Autodesk Inventor part; units mm, degrees
ref_plane "YZ Plane" through (0, 0, 0) normal (1, 0, 0) x (0, 1, 0)
ref_plane "XZ Plane" through (0, 0, 0) normal (0, 1, 0) x (-1, 0, 0)
ref_plane "XY Plane" through (0, 0, 0) normal (0, 0, 1) x (1, 0, 0)
sketch "Esquisse1" plane through (0, 0, 0) normal (0, 1, 0) x (-1, 0, 0)
  line L0 (-32.5, 48.5) -> (32.5, 48.5)
  line L1 (32.5, 48.5) -> (32.5, -48.5)
  line L2 (32.5, -48.5) -> (-32.5, -48.5)
  line L3 (-32.5, -48.5) -> (-32.5, 48.5)
  point P0 (0, 0)
  dimension "d0" = 65
  dimension "d1" = 97
  dimension "d2" = 32.5
  dimension "d3" = 48.5
extrude "Extrusion1" add sketch "Esquisse1" along normal blind 1.5
sketch "Esquisse2" plane through (0, 1.5, 0) normal (0, 1, 0) x (1, 0, 0)
  line L0 (-32.5, -48.5) -> (32.5, -48.5)
  line L1 (32.5, -48.5) -> (32.5, 48.5)
  line L2 (-32.5, 48.5) -> (-32.5, -48.5)
  line L3 (-27.5, 17.5) -> (-22.5, 17.5)
  line L4 (-22.5, 17.5) -> (-22.5, -47.5)
  line L5 (-22.5, -47.5) -> (-27.5, -47.5)
  line L6 (-27.5, -47.5) -> (-27.5, 17.5)
  line L7 (22.5, 17.5) -> (27.5, 17.5)
  line L8 (27.5, 17.5) -> (27.5, -47.5)
  line L9 (27.5, -47.5) -> (22.5, -47.5)
  line L10 (22.5, -47.5) -> (22.5, 17.5)
  point P0 (0, 0)
  dimension "d6" = 5
  dimension "d7" = 5
  dimension "d8" = 65
  dimension "d9" = 5
  dimension "d10" = 5
  dimension "d11" = 1
extrude "Extrusion2" add sketch "Esquisse2" along normal blind 9 and the other way blind 5.5
sketch "Esquisse3" plane through (0, 0, 0) normal (0, -1, 0) x (1, 0, 0)
  line L0 (32.5, 48.5) -> (-32.5, 48.5)
  line L1 (32.5, -48.5) -> (32.5, 48.5)
  line L2 (9.5, 48.5) -> (17.5, 48.5)
  line L3 (17.5, 48.5) -> (17.5, 33.5)
  line L4 (17.5, 33.5) -> (9.5, 33.5)
  line L5 (9.5, 33.5) -> (9.5, 48.5)
  point P0 (0, 0)
  dimension "d16" = 15
  dimension "d17" = 8
  dimension "d18" = 15
extrude "Extrusion3" add sketch "Esquisse3" along normal blind 14
sketch "Esquisse4" plane through (-32.5, 1.5, 48.5) normal (0, 0, 1) x (1, 0, 0)
  line L0 (50, -15.5) -> (42, -15.5)
  line L1 (50, -1.5) -> (50, -15.5)
  circle A0 centre (47, -10.5) radius 2.5
  point P0 (32.5, -1.5)
  dimension "d21" = 5
  dimension "d22" = 5
  dimension "d23" = 3
extrude "Extrusion4" add sketch "Esquisse4" along normal blind 4
sketch "Esquisse5" plane through (0, 0, 0) normal (0, -1, 0) x (1, 0, 0)
  line L0 (9.5, 48.5) -> (-32.5, 48.5)
  line L1 (-32.5, 48.5) -> (-32.5, -48.5)
  line L2 (32.5, -48.5) -> (32.5, 48.5)
  line L3 (32.5, 48.5) -> (17.5, 48.5)
  circle A0 centre (-12.5, 18.5) radius 2.5
  circle A1 centre (12.5, 18.5) radius 2.5
  point P0 (0, 0)
  dimension "d26" = 30
  dimension "d27" = 30
  dimension "d28" = 25
  dimension "d29" = 20
  dimension "d30" = 65
  dimension "d31" = 5
  dimension "d32" = 5
extrude "Extrusion5" add sketch "Esquisse5" along normal blind 10
sketch "Esquisse6" plane through (0, 0, 0) normal (0, -1, 0) x (1, 0, 0)
  line L0 (-32.5, 48.5) -> (-32.5, -48.5)
  line L1 (-32.5, -48.5) -> (32.5, -48.5)
  line L2 (32.5, -48.5) -> (32.5, 48.5)
  line L3 (27.5, -17.5) -> (22.5, -17.5)
  line L4 (22.5, -17.5) -> (22.5, 47.5)
  line L5 (25, -23.5) -> (27.5, -23.5)
  line L6 (27.5, -23.5) -> (27.5, -38.5)
  line L7 (27.5, -38.5) -> (25, -38.5)
  line L8 (25, -38.5) -> (25, -23.5)
  line L9 (-15.5, -23.5) -> (-13, -23.5)
  line L10 (-13, -23.5) -> (-13, -33.5)
  line L11 (-13, -33.5) -> (-15.5, -33.5)
  line L12 (-15.5, -33.5) -> (-15.5, -23.5)
  line L13 (14, -5) -> (16.5, -5)
  line L14 (16.5, -5) -> (16.5, -10)
  line L15 (16.5, -10) -> (14, -10)
  line L16 (14, -10) -> (14, -5)
  point P0 (0, 0)
  dimension "d35" = 2.5
  dimension "d36" = 2.5
  dimension "d37" = 2.5
  dimension "d38" = 10
  dimension "d39" = 5
  dimension "d40" = 15
  dimension "d41" = 5
  dimension "d42" = 17
  dimension "d43" = 6
  dimension "d44" = 10
  dimension "d45" = 15
  dimension "d46" = 7.5
extrude "Extrusion6" add sketch "Esquisse6" along normal blind 8
sketch "Esquisse7" plane through (0, 0, 0) normal (0, -1, 0) x (1, 0, 0)
  line L0 (-32.5, 48.5) -> (-32.5, -48.5)
  line L1 (-32.5, -48.5) -> (32.5, -48.5)
  line L2 (-4, -40.5) -> (4, -40.5)
  line L3 (4, -40.5) -> (4, -50.5)
  line L4 (4, -50.5) -> (-4, -50.5)
  line L5 (-4, -50.5) -> (-4, -40.5)
  point P0 (0, 0)
  dimension "d49" = 10
  dimension "d50" = 8
  dimension "d51" = 65
  dimension "d52" = 28.5
  dimension "d53" = 2
extrude "Extrusion7" add sketch "Esquisse7" along normal blind 3.5
sketch "Esquisse8" plane through (0, 1.5, 0) normal (0, 1, 0) x (1, 0, 0)
  line L0 (32.5, -48.5) -> (32.5, 48.5)
  line L1 (32.5, 48.5) -> (-32.5, 48.5)
  line L2 (-32.5, 48.5) -> (-32.5, -48.5)
  line L3 (-27.5, 46.5) -> (-25, 46.5)
  line L4 (-25, 46.5) -> (-25, 41.5)
  line L5 (-25, 41.5) -> (-27.5, 41.5)
  line L6 (-27.5, 41.5) -> (-27.5, 46.5)
  line L7 (25, 46.5) -> (27.5, 46.5)
  line L8 (27.5, 46.5) -> (27.5, 41.5)
  line L9 (27.5, 41.5) -> (25, 41.5)
  line L10 (25, 41.5) -> (25, 46.5)
  point P0 (0, 0)
  dimension "d56" = 2.5
  dimension "d57" = 2.5
  dimension "d58" = 5
  dimension "d59" = 5
  dimension "d60" = 2
  dimension "d61" = 2
  dimension "d62" = 5
  dimension "d63" = 5
extrude "Extrusion8" add sketch "Esquisse8" along normal blind 9
equation "\"d7\" = d6"
equation "\"d9\" = d6"
equation "\"d10\" = d9"
equation "\"d27\" = d26"
equation "\"d29\" = -0.5 * d28 + 0.5 * d30"
equation "\"d32\" = d31"
equation "\"d52\" = -0.5 * d50 + 0.5 * d51"
equation "\"d57\" = d56"
equation "\"d61\" = d60"
equation "\"d63\" = d62"
properties part number "discovery"
Input: part model. Units: mm. Frame: model coordinates. A direction names the side the tool comes from. Give positions to 0.01 mm unless a question says otherwise; leave off trailing zeros. Order: outer loops, then holes, each group sorted by start corner. A loop starts at its lowest first (then second) coordinate and runs counter-clockwise, first axis right, second up. Notation, with made-up numbers: (-0.75, 82) - (52.25, 82) arc R30 ccw to (52.25, 121) - close; hole circle Ø4 at (26.25, -18.5). An arc over 180 degrees is marked (long way). One line per item, written item: value.
1. Cut plane A-A, the plane y = -9. Output: boundary loops of the cut face in (x, z), and give its area (3 significant figures).
Determined:
outline: circle Ø5 at (-12.5, 18.5); (9.5, 33.5) - (17.5, 33.5) - (17.5, 48.5) - (17, 48.5) - (17, 52.5) - (12, 52.5) - (12, 48.5) - (9.5, 48.5) - close; circle Ø5 at (12.5, 18.5)
area: 179 mm2
2. Cut plane C-C, the plane z = 1.5. Output: boundary loops of the cut face in (x, y).
Determined:
outline: (-32.5, 0) - (-27.5, 0) - (-27.5, -4) - (-22.5, -4) - (-22.5, 0) - (22.5, 0) - (22.5, -4) - (27.5, -4) - (27.5, 0) - (32.5, 0) - (32.5, 1.5) - (27.5, 1.5) - (27.5, 10.5) - (22.5, 10.5) - (22.5, 1.5) - (-22.5, 1.5) - (-22.5, 10.5) - (-27.5, 10.5) - (-27.5, 1.5) - (-32.5, 1.5) - close
3. Draft query along Z for faces 1 (the face through (14, -9, 52.5)), 2 (the face through (0, 0, -49)), 3 (the face through (10, -4.9, 18.4)). Return one class per face: released by +Z, released by -Z, zero draft, split by the parting line, or undercut.
Determined:
face 1: released by +Z
face 2: zero draft
face 3: undercut
4. Cut plane B-B, the plane x = 24. Output: boundary loops of the cut face in (y, z).
Determined:
outline: (-4, -17.5) - (0, -17.5) - (0, -48.5) - (1.5, -48.5) - (1.5, -17.5) - (10.5, -17.5) - (10.5, 47.5) - (1.5, 47.5) - (1.5, 48.5) - (0, 48.5) - (0, 47.5) - (-4, 47.5) - close
5. Cut plane D-D, the plane z = 43. Output: boundary loops of the cut face in (x, y), and give its area (4 significant figures).
Determined:
outline: (-32.5, 0) - (-27.5, 0) - (-27.5, -4) - (-22.5, -4) - (-22.5, 0) - (9.5, 0) - (9.5, -14) - (17.5, -14) - (17.5, 0) - (22.5, 0) - (22.5, -4) - (27.5, -4) - (27.5, 0) - (32.5, 0) - (32.5, 1.5) - (27.5, 1.5) - (27.5, 10.5) - (22.5, 10.5) - (22.5, 1.5) - (-22.5, 1.5) - (-22.5, 10.5) - (-27.5, 10.5) - (-27.5, 1.5) - (-32.5, 1.5) - close
area: 339.5 mm2
6. Pin query (flat end, axial travel): pin 1 Ø2 at (x, y) = (-26, 4) entering from -Z; pin 2 Ø0.8 at (x, y) = (3, 0.5) entering from -Z; pin 3 Ø1.2 at (x, z) = (26.5, -33) entering from -Y. Return the tip coordinate at first contact, or that it passes through.
Determined:
pin 1: z = -46.5
pin 2: z = -48.5
pin 3: y = -8
7. Line query: probe 1 along X at (y, z) = (4, -8); probe 2 along X at (y, z) = (-3.25, -25); probe 3 along X at (y, z) = (-9.25, 40.5). Output: solid intervals per line, ascending.
Determined:
probe 1: -27.5 to -22.5, 22.5 to 27.5
probe 2: -15.5 to -13, 25 to 27.5
probe 3: 9.5 to 17.5
8. Reachability of faces 4 (the face through (25, 6, -44)), 5 (the face through (-25, 6, 47.5)), 6 (the face through (-27.5, -2, 15)), 7 (the face through (15, -4, -5)) from +Z, -Z, +X, -X, +Y, -Y: full face, straight path, thin tool, end or side. Return the list, or none.
Determined:
face 4: -Z, +Y
face 5: +Z, +X, -X, +Y
face 6: +Z, -Z, -X, -Y
face 7: -Y
